from build123d import *

# Parameters (mm, degrees)
SKETCH1_W           = 49
SKETCH1_H           = 75
BOSS_EXTRUDE1_DEPTH = 3.2
CUT_EXTRUDE1_REACH  = 5.2
SKETCH2_R           = 20.445


with BuildPart() as part:
    # Sketch1 → Boss-Extrude1 (new body)
    with BuildSketch(Plane(origin=(0, 0, 0), x_dir=(0, 0, -1), z_dir=(1, 0, 0))):
        with Locations((24.5, 37.5)):
            Rectangle(SKETCH1_W, SKETCH1_H)
    extrude(amount=BOSS_EXTRUDE1_DEPTH)

    # Sketch2 → Cut-Extrude1 (cut, up to next)
    with BuildSketch(Plane(origin=(3.2, 0, 0), x_dir=(0, 0, -1), z_dir=(1, 0, 0)), mode=Mode.PRIVATE) as cut_extrude1_sk1:
        with Locations((24.5, 45.495825453)):
            Circle(SKETCH2_R)
    cut_extrude1_tool1 = extrude(cut_extrude1_sk1.sketch, amount=-CUT_EXTRUDE1_REACH, mode=Mode.PRIVATE) & part.part
    add(cut_extrude1_tool1.solids().sort_by_distance((3.2, 45.495825, -24.5))[0], mode=Mode.SUBTRACT)


solid = part.part
Read the model definition and answer for the solid it produces. Units are mm, in the model's axes. Give positions to 0.01 mm unless a question says otherwise; leave off trailing zeros. Write each loop counter-clockwise with the first axis right and the second up, starting at its lowest first coordinate (ties: lowest second). Pieces come first, ordered by that corner, then holes. Notation, with made-up numbers: (-13, 41.5) - (26, 41.5) arc R14 ccw to (26, 52.5) - close; hole circle Ø10 at (67, -27). An arc over 180 degrees is marked (long way). Answer in a Markdown table with one row per item. Add a question column.
Item 1: Section B-B, the plane y = 26.5 is taken. Write down the section's boundary in (x, z), and give its area (3 significant figures).
Item 2: Find the intervals of material crossed by L1, parallel to Y at x = 0.6, z = -24.5; L2, parallel to Z at x = 1.05, y = 61; L3, parallel to Z at x = 2.4, y = 46, in increasing order.
Item 3: Section C-C, the plane x = 2.3 is taken. Write down the section's boundary in (y, z) (3 decimals).
Item 4: Determine the mould class of faces 1 (the face through (0, 21, -24)), 2 (the face through (1.622, 27.358, -33.934)), 3 (the face through (2, 75, -24)), 4 (the face through (2, 0, -24)) for opening direction Y: pulls with the +Y half, pulls with the -Y half, needs draft (parallel to the pull), parting line crosses it, or undercut.
Item 5: Section A-A, the plane z = -24.5 is taken. Write down the section's boundary in (x, y), and give its area (3 significant figures).
Item 6: A flat-ended cylindrical pin translates along its axis: P1, Ø10, axis at y = 30.5, z = -12.5, coming from the -X side. Find the tip coordinate at first contact, or state that the pin passes through.
Recorded:
| question | item | result |
|---|---|---|
| 1 | outline | (0, -49) - (3.2, -49) - (3.2, -32.06) - (0, -32.06) - close; (0, -16.94) - (3.2, -16.94) - (3.2, 0) - (0, 0) - close |
| 1 | area | 108 mm2 |
| 2 | L1 | y = 0 to 25.05, 65.94 to 75 |
| 2 | L2 | z = -49 to -37.83, -11.17 to 0 |
| 2 | L3 | z = -49 to -44.94, -4.06 to 0 |
| 3 | outline | (0, -49) - (75, -49) - (75, 0) - (0, 0) - close; hole circle Ø40.89 at (45.496, -24.5) |
| 4 | face 1 | needs draft |
| 4 | face 2 | undercut |
| 4 | face 3 | pulls with the +Y half |
| 4 | face 4 | pulls with the -Y half |
| 5 | outline | (0, 0) - (3.2, 0) - (3.2, 25.05) - (0, 25.05) - close; (0, 65.94) - (3.2, 65.94) - (3.2, 75) - (0, 75) - close |
| 5 | area | 109 mm2 |
| 6 | P1 | stops at x = 0 |
